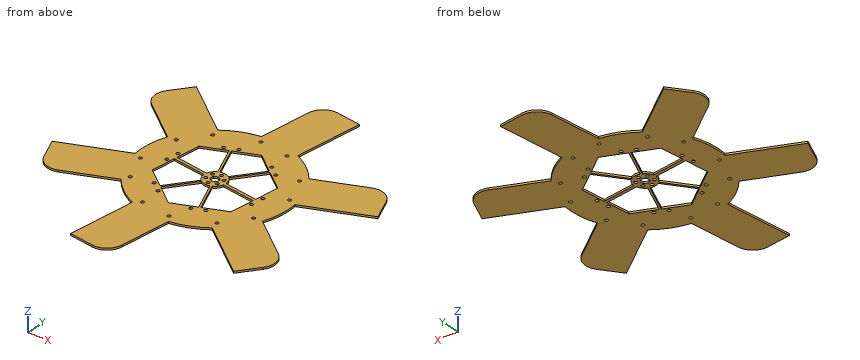
```python
from build123d import *

# Parameters (mm, degrees)
SKETCH1_R            = 127
BOSS_EXTRUDE1_DEPTH  = 3.175
M5_CLEARANCE_HOLE1_D = 5.5
CIRPATTERN1_COUNT    = 6
BOSS_EXTRUDE2_DEPTH  = 3.175
CIRPATTERN2_COUNT    = 6
CUT_EXTRUDE1_REACH   = 335.168
CUT_EXTRUDE2_DEPTH   = 334.167593846


with BuildPart() as part:
    # Sketch1 → Boss-Extrude1 (new body)
    with BuildSketch(Plane.XY):
        Circle(SKETCH1_R)
    extrude(amount=BOSS_EXTRUDE1_DEPTH)

    # M5 Clearance Hole1 (through all)
    with Locations(Plane(origin=(0, 0, 0), x_dir=(-1, 0, 0), z_dir=(0, 0, -1))):
        with Locations((-58.2494214, 58.493652703), (-82.549819355, -0.172697611), (-93.238867767, 66.113565457), (-112.679186132, 19.180485205), (-11.733270063, 4.860079591)):
            m5_clearance_hole1 = Hole(M5_CLEARANCE_HOLE1_D / 2)

    # CirPattern1: M5 Clearance Hole1 ×6 about axis
    cirpattern1_axis = Axis((-0.168463788, -0.069779986, 0), (0, 0, 1))
    for i in range(1, CIRPATTERN1_COUNT):
        add(m5_clearance_hole1.rotate(cirpattern1_axis, i * 360 / CIRPATTERN1_COUNT), mode=Mode.SUBTRACT)

    # Sketch6 → Boss-Extrude2 (add)
    with BuildSketch(Plane(origin=(0, 0, 0), x_dir=(-1, 0, 0), z_dir=(0, 0, -1))):
        with BuildLine():
            Line((-92.527543442, 76.128710982), (-180.527068914, 112.579307915))
            ThreePointArc((-180.527068914, 112.579307915), (-202.397427074, 112.579307915), (-217.862105635, 97.114629353))
            Line((-217.862105635, 97.114629353), (-233.657364306, 58.981501649))
            Line((-233.657364306, 58.981501649), (-119.257981193, 11.595725636))
            Line((-119.257981193, 11.595725636), (-92.527543442, 76.128710982))
        make_face()
    boss_extrude2 = extrude(amount=-BOSS_EXTRUDE2_DEPTH)

    # CirPattern2: Boss-Extrude2 ×6 about axis
    cirpattern2_axis = Axis((0, 0, 0), (0, 0, 1))
    for i in range(1, CIRPATTERN2_COUNT):
        add(boss_extrude2.rotate(cirpattern2_axis, i * 360 / CIRPATTERN2_COUNT))

    # Sketch7 → Cut-Extrude1 (cut, up to next)
    with BuildSketch(Plane.XY, mode=Mode.PRIVATE) as cut_extrude1_sk1:
        with BuildLine():
            Line((-30.627136304, 69.792110428), (-69.805717322, 53.563810816))
            Line((-69.805717322, 53.563810816), (-75.223541932, 12.411347252))
            Line((-75.223541932, 12.411347252), (-18.400886991, 4.930502809))
            ThreePointArc((-18.400886991, 4.930502809), (-14.833899914, 11.952318325), (-8.731421131, 16.931177899))
            Line((-8.731421131, 16.931177899), (-30.627136304, 69.792110428))
        make_face()
    cut_extrude1_tool1 = extrude(cut_extrude1_sk1.sketch, amount=CUT_EXTRUDE1_REACH, mode=Mode.PRIVATE) & part.part
    # Sketch7 → Cut-Extrude1 (cut, up to next)
    with BuildSketch(Plane.XY, mode=Mode.PRIVATE) as cut_extrude1_sk2:
        with BuildLine():
            Line((81.290479551, 33.671619122), (47.647069318, 59.487115762))
            Line((47.647069318, 59.487115762), (12.816016466, 14.094403923))
            ThreePointArc((12.816016466, 14.094403923), (17.421934647, 7.705757144), (19.05, 0))
            Line((19.05, 0), (75.872654941, -7.480844443))
            Line((75.872654941, -7.480844443), (81.290479551, 33.671619122))
        make_face()
    cut_extrude1_tool2 = extrude(cut_extrude1_sk2.sketch, amount=CUT_EXTRUDE1_REACH, mode=Mode.PRIVATE) & part.part
    # Sketch7 → Cut-Extrude1 (cut, up to next)
    with BuildSketch(Plane.XY, mode=Mode.PRIVATE) as cut_extrude1_sk3:
        with BuildLine():
            Line((11.484762229, 87.235429938), (-27.693818788, 71.007130326))
            Line((-27.693818788, 71.007130326), (-5.798103615, 18.146197797))
            ThreePointArc((-5.798103615, 18.146197797), (2.486523962, 18.887024609), (10.297119611, 16.02722146))
            Line((10.297119611, 16.02722146), (45.128172463, 61.419933299))
            Line((45.128172463, 61.419933299), (11.484762229, 87.235429938))
        make_face()
    cut_extrude1_tool3 = extrude(cut_extrude1_sk3.sketch, amount=CUT_EXTRUDE1_REACH, mode=Mode.PRIVATE) & part.part
    # Sketch7 → Cut-Extrude1 (cut, up to next)
    with BuildSketch(Plane.XY, mode=Mode.PRIVATE) as cut_extrude1_sk4:
        with BuildLine():
            Line((-81.290479551, -33.671619122), (-47.647069318, -59.487115762))
            Line((-47.647069318, -59.487115762), (-12.816016466, -14.094403923))
            ThreePointArc((-12.816016466, -14.094403923), (-17.421934647, -7.705757144), (-19.05, 0))
            Line((-19.05, 0), (-75.872654941, 7.480844443))
            Line((-75.872654941, 7.480844443), (-81.290479551, -33.671619122))
        make_face()
    cut_extrude1_tool4 = extrude(cut_extrude1_sk4.sketch, amount=CUT_EXTRUDE1_REACH, mode=Mode.PRIVATE) & part.part
    # Sketch7 → Cut-Extrude1 (cut, up to next)
    with BuildSketch(Plane.XY, mode=Mode.PRIVATE) as cut_extrude1_sk5:
        with BuildLine():
            Line((-11.484762229, -87.235429938), (27.693818788, -71.007130326))
            Line((27.693818788, -71.007130326), (5.798103615, -18.146197797))
            ThreePointArc((5.798103615, -18.146197797), (-2.486523962, -18.887024609), (-10.297119611, -16.02722146))
            Line((-10.297119611, -16.02722146), (-45.128172463, -61.419933299))
            Line((-45.128172463, -61.419933299), (-11.484762229, -87.235429938))
        make_face()
    cut_extrude1_tool5 = extrude(cut_extrude1_sk5.sketch, amount=CUT_EXTRUDE1_REACH, mode=Mode.PRIVATE) & part.part
    # Sketch7 → Cut-Extrude1 (cut, up to next)
    with BuildSketch(Plane.XY, mode=Mode.PRIVATE) as cut_extrude1_sk6:
        with BuildLine():
            Line((69.805717322, -53.563810816), (75.223541932, -12.411347252))
            Line((75.223541932, -12.411347252), (18.400886991, -4.930502809))
            ThreePointArc((18.400886991, -4.930502809), (14.833899914, -11.952318325), (8.731421131, -16.931177899))
            Line((8.731421131, -16.931177899), (30.627136304, -69.792110428))
            Line((30.627136304, -69.792110428), (69.805717322, -53.563810816))
        make_face()
    cut_extrude1_tool6 = extrude(cut_extrude1_sk6.sketch, amount=CUT_EXTRUDE1_REACH, mode=Mode.PRIVATE) & part.part
    add(cut_extrude1_tool1.solids().sort_by_distance((-43.105306, 33.563643, 0))[0], mode=Mode.SUBTRACT)
    add(cut_extrude1_tool2.solids().sort_by_distance((50.323438, 21.263515, 0))[0], mode=Mode.SUBTRACT)
    add(cut_extrude1_tool3.solids().sort_by_distance((7.102658, 53.950047, 0))[0], mode=Mode.SUBTRACT)
    add(cut_extrude1_tool4.solids().sort_by_distance((-50.323438, -21.263515, 0))[0], mode=Mode.SUBTRACT)
    add(cut_extrude1_tool5.solids().sort_by_distance((-7.102658, -53.950047, 0))[0], mode=Mode.SUBTRACT)
    add(cut_extrude1_tool6.solids().sort_by_distance((43.105306, -33.563643, 0))[0], mode=Mode.SUBTRACT)

    # Sketch16 → Cut-Extrude2 (cut, through all)
    with BuildSketch(Plane.XY.offset(3.175)):
        Polygon((6.774206629, 2.80596826), (0.957063519, 7.269619162), (-5.81714311, 4.463650901), (-6.774206629, -2.80596826), (-0.957063519, -7.269619162), (5.81714311, -4.463650901), align=None)
    extrude(amount=-CUT_EXTRUDE2_DEPTH, mode=Mode.SUBTRACT)


solid = part.part
```
Check sheet for the modelled part. Datum: model origin and axes. Units: mm. Round coordinates to 2 decimals unless told otherwise and drop trailing zeros. Order: outer loops, then holes, each group sorted by start corner. A loop starts at its lowest first (then second) coordinate and runs counter-clockwise, first axis right, second up.
1) Section check A-A (x = -160). Record the boundary of the cut face in (y, z) (3 decimals), and give its area (3 significant figures).
2) Go/stop test with flat-tipped pins: pin 1 Ø5 at (x, y) = (10.05, -7.91) entering from +Z; pin 2 Ø1 at (y, z) = (104, 2) entering from +X; pin 3 Ø1.5 at (y, z) = (-88, 1) entering from -X. Record where each tip stops, or that it passes through.
3) Scan lines: line 1 (Y direction, x = 50, z = 1.7); line 2 (X direction, y = -71, z = 1.25); line 3 (X direction, y = 109, z = 0.75) (3 decimals). Record each from-to range of solid material in increasing order.
4) Section check B-B (z = 1.95). Give the number of separate pieces and of enclosed holes in the cut face, and give its area (3 significant figures).
Result:
1. outline: (-104.077, 0) - (-28.472, 0) - (-28.472, 3.175) - (-104.077, 3.175) - close; (78.75, 0) - (166.794, 0) - (166.794, 3.175) - (78.75, 3.175) - close
1. area: 520 mm2
2. pin 1: passes through
2. pin 2: stops at x = 214.19
2. pin 3: stops at x = -221.95
3. line 1: y = -116.74 to -61.77, -9.09 to -4.07, 57.68 to 233.92
3. line 2: x = -228.68 to -44.29, -38.95 to -32.64, 27.69 to 38.46, 43.75 to 149.9
3. line 3: x = -195.43 to -84.681, -65.177 to 37.435, 41.733 to 65.177, 171.886 to 208.66
4. separate pieces: 1
4. enclosed holes: 37
4. area: 78,500 mm2
